```python
from build123d import *

# Parameters (mm, degrees)
BOSS_EXTRUDE1_DEPTH     = 10
SKETCH3_W               = 27
SKETCH3_H               = 4
BOSS_EXTRUDE2_DEPTH     = 17
SKETCH4_R               = 1.5
CUT_EXTRUDE1_DEPTH      = 4
CUT_EXTRUDE2_DEPTH      = 15
CUT_EXTRUDE2_DEPTH_BACK = 27
SKETCH5_W               = 24.801401456
SKETCH5_H               = 70.149949376


with BuildPart() as part:
    # Sketch1 → Boss-Extrude1 (new body)
    with BuildSketch(Plane.XY):
        with BuildLine():
            Line((0.947795447, 55.867567374), (-5.354013975, 64.102890964))
            ThreePointArc((-5.354013975, 64.102890964), (-14.235235054, 34.948420067), (0, 8))
            Line((0, 8), (0, 4))
            Line((0, 4), (0, 0))
            Line((0, 0), (27, 0))
            Line((27, 0), (27, 4))
            Line((27, 4), (12, 4))
            Line((12, 4), (12, 12))
            ThreePointArc((12, 12), (-3.507060252, 31.419133439), (0.947795447, 55.867567374))
        make_face()
    boss_extrude1 = extrude(amount=BOSS_EXTRUDE1_DEPTH)

    # Sketch3 → Boss-Extrude2 (add)
    with BuildSketch(Plane.XY):
        with Locations((13.5, 2)):
            Rectangle(SKETCH3_W, SKETCH3_H)
    boss_extrude2 = extrude(amount=BOSS_EXTRUDE2_DEPTH)

    # Sketch4 → Cut-Extrude1 (cut)
    with BuildSketch(Plane(origin=(0, 4, 0), x_dir=(1, 0, 0), z_dir=(0, 1, 0))):
        with Locations(Location((5, -13, 0), (0, 0, 270))):
            Circle(SKETCH4_R)
        with Locations(Location((11, -13, 0), (0, 0, 270))):
            Circle(SKETCH4_R)
        with Locations(Location((17, -13, 0), (0, 0, 270))):
            Circle(SKETCH4_R)
        with Locations(Location((23, -13, 0), (0, 0, 270))):
            Circle(SKETCH4_R)
    cut_extrude1 = extrude(amount=-CUT_EXTRUDE1_DEPTH, mode=Mode.SUBTRACT)

    # Mirror8: Boss-Extrude1, Boss-Extrude2, Cut-Extrude1 across plane
    add(boss_extrude1.mirror(Plane(origin=(27, 0, 10), x_dir=(0, 0, 1), z_dir=(-1, 0, 0))))
    add(boss_extrude2.mirror(Plane(origin=(27, 0, 10), x_dir=(0, 0, 1), z_dir=(-1, 0, 0))))
    add(cut_extrude1.mirror(Plane(origin=(27, 0, 10), x_dir=(0, 0, 1), z_dir=(-1, 0, 0))), mode=Mode.SUBTRACT)

    # Sketch5 → Cut-Extrude2 (cut, two sides: drawn at the far end of the back side and taken through both)
    with BuildSketch(Plane.ZY.offset(-CUT_EXTRUDE2_DEPTH_BACK)):
        with Locations((8.5, 31.779897291)):
            Rectangle(SKETCH5_W, SKETCH5_H)
    extrude(amount=CUT_EXTRUDE2_DEPTH + CUT_EXTRUDE2_DEPTH_BACK, mode=Mode.SUBTRACT)


solid = part.part
```
For this review, take the finished solid that the model builds, in its own axes (mm). A direction names the side the tool comes from. Coordinates: 2 decimals unless noted, no trailing zeros. Loops run counter-clockwise (first coordinate to the right, second up) from the corner with the lowest first, then second, coordinate; pieces in that order, holes last. Notation, with made-up numbers: (8.25, -12.75) -> (51.25, -12.75) arc R28 cw to (51.25, 24.25) -> close; hole circle Ø3 at (-6, 26). An arc over 180 degrees is marked (long way). Return JSON: item names as keys, results as strings. Group by question number.
(1) To check wall thickness, follow L1, parallel to X at y = 1.3, z = 13; L2, parallel to Z at x = 49, y = 2; L3, parallel to Y at x = 45, z = 12. State the ranges of each line that lie inside material, in increasing order.
(2) Mouldability with a two-part tool opening along Z and no side actions: class faces 1 (the cylindrical face through (50.464, 2.028, 12.675)), 2 (the cylindrical face through (44.464, 2.028, 12.675)), 3 (the flat face through (41, 2, 17)), 4 (the flat face through (56.16, 59.93, 4.93)) as pulls with the +Z half, pulls with the -Z half, needs draft (parallel to the pull), parting line crosses it, or undercut.
(3) Consider section A-A, the plane x = 31. Give the boundary of the cut face in (y, z).
(4) Tool access review of faces 5 (the flat face through (54, 3, 6)), 6 (the flat face through (58.3, 34.5, 10)), 7 (the cylindrical face through (38.464, 2.028, 12.675)), 8 (the flat face through (42, 8, 5)), 9 (the cylindrical face through (57.417, 31.072, 4.93)): name each direction out of +Z, -Z, +X, -X, +Y, -Y from which nothing blocks a thin tool from reaching the whole face with its end or side.
(5) For pin 1 Ø8 at (y, z) = (39.5, 3) entering from -X; pin 2 Ø4 at (x, z) = (31, 13) entering from +Y; pin 3 Ø6.5 at (y, z) = (7.5, 4) entering from -X; pin 4 Ø2.5 at (x, z) = (43, 13) entering from -Y, all flat-tipped, find the tip position at first contact; note any pin that passes through.
(6) Consider section C-C, the plane x = 43. Give the boundary of the cut face in (y, z), plus the area to 3 significant figures.
(7) Consider section B-B, the plane z = 4.5. Give the boundary of the cut face in (x, y), plus the area to 3 significant figures.
(8) Consider section D-D, the plane y = 27. Give the boundary of the cut face in (x, z), plus the area to 3 significant figures.
Results below:
{
 "1": {"L1": "x = 27 to 29.5, 32.5 to 35.5, 38.5 to 41.5, 44.5 to 47.5, 50.5 to 54", "L2": "z = 0 to 11.5, 14.5 to 17", "L3": "y = 0 to 4"},
 "2": {"face 1": "undercut", "face 2": "undercut", "face 3": "pulls with the +Z half", "face 4": "needs draft"},
 "3": {"outline": "(0, 0) -> (4, 0) -> (4, 11.5) -> (0, 11.5) -> close; (0, 14.5) -> (4, 14.5) -> (4, 17) -> (0, 17) -> close"},
 "4": {"face 5": "+Z, -Z, +X, -Y", "face 6": "+Z, +X, -X, +Y", "face 7": "+Y, -Y", "face 8": "+Z, -Z, -X, +Y", "face 9": "+Z, -Z, -X"},
 "5": {"pin 1": "stops at x = 58.04", "pin 2": "stops at y = 4", "pin 3": "stops at x = 42", "pin 4": "passes through"},
 "6": {"outline": "(0, 0) -> (12.53, 0) -> (12.53, 10) -> (4, 10) -> (4, 11.5) -> (0, 11.5) -> close; (0, 14.5) -> (4, 14.5) -> (4, 17) -> (0, 17) -> close", "area": "141 mm2"},
 "7": {"outline": "(27, 0) -> (54, 0) -> (54, 8) arc R40 ccw to (59.35, 64.1) -> (53.05, 55.87) arc R30 cw to (42, 12) -> (42, 4) -> (27, 4) -> close", "area": "748 mm2"},
 "8": {"outline": "(56.02, 0) -> (66.65, 0) -> (66.65, 10) -> (56.02, 10) -> close", "area": "106 mm2"}
}
